```python
from build123d import *

# Parameters (mm, degrees)
BOSS_EXTRUDE1_DEPTH      = 30
SKETCH3_R                = 2.146244949
BOSS_EXTRUDE2_DEPTH      = 10
BOSS_EXTRUDE2_DEPTH_BACK = 104
SKETCH4_W                = 62.472603167
SKETCH4_H                = 24.76734243
CUT_EXTRUDE1_DEPTH       = 31
FILLET1_R                = 10
SKETCH5_R                = 0.76292284
BOSS_EXTRUDE3_DEPTH      = 30
SKETCH8_W                = 88.333137
SKETCH8_H                = 25.902143048
CUT_EXTRUDE2_DEPTH       = 5
SKETCH9_R                = 0.25
BOSS_EXTRUDE4_DEPTH      = 90


with BuildPart() as part:
    # Sketch1 → Boss-Extrude1 (new body)
    with BuildSketch(Plane(origin=(0, 0, 0), x_dir=(1, 0, 0), z_dir=(0, 1, 0))):
        Polygon((-80.330769327, 39.448145651), (-80.330769327, -54.366717098), (84.060412188, -54.366717098), (125.94717048, -7.459285723), (76.88802207, 39.448145651), align=None)
    extrude(amount=BOSS_EXTRUDE1_DEPTH)

    # Sketch2 → Cut-Revolve2 (revolve, cut)
    with BuildSketch(Plane(origin=(73.778167937, 0, 65.881422133), x_dir=(0.666061097, 0, -0.745897188), z_dir=(0.745897188, 0, 0.666061097))):
        with BuildLine():
            Line((32.647209403, 24.725169295), (66.605654017, 24.725169295))
            ThreePointArc((66.605654017, 24.725169295), (77.035151749, 14.295671563), (66.605654017, 3.866173832))
            Line((66.605654017, 3.866173832), (32.647209403, 3.866173832))
            ThreePointArc((32.647209403, 3.866173832), (22.217711672, 14.295671563), (32.647209403, 24.725169295))
        make_face()
    revolve(axis=Axis((125.94717048, 30, 7.459285723), (0, -1, 0)), mode=Mode.SUBTRACT)

    # Sketch3 → Boss-Extrude2 (add, two sides)
    with BuildSketch(Plane.XY.offset(54.366717098)) as boss_extrude2_sk:
        with Locations((-57.321321229, 15)):
            Circle(SKETCH3_R)
    extrude(amount=BOSS_EXTRUDE2_DEPTH)
    extrude(boss_extrude2_sk.sketch, amount=-BOSS_EXTRUDE2_DEPTH_BACK)

    # Sketch4 → Cut-Extrude1 (cut, through all)
    with BuildSketch(Plane(origin=(0, 30, 0), x_dir=(1, 0, 0), z_dir=(0, 1, 0))):
        with Locations((145.25317231, -8.435915945)):
            Rectangle(SKETCH4_W, SKETCH4_H)
    extrude(amount=-CUT_EXTRUDE1_DEPTH, mode=Mode.SUBTRACT)

    # Fillet1
    fillet1_edges = [part.edges().sort_by_distance(p)[0] for p in [
        (114.016870726, 1.933086916, 20.81958716),
        (114.016870726, 27.362584647, 20.81958716),
        (114.016870726, 1.933086916, -3.94775527),
        (114.016870726, 27.362584647, -3.94775527),
    ]]
    fillet(fillet1_edges, radius=FILLET1_R)

    # Sketch5 → Boss-Extrude3 (add)
    with BuildSketch(Plane(origin=(0, 30, 0), x_dir=(1, 0, 0), z_dir=(0, 1, 0))):
        with Locations((109.099187599, -8.665449149)):
            Circle(SKETCH5_R)
    extrude(amount=-BOSS_EXTRUDE3_DEPTH)

    # Sketch8 → Cut-Extrude2 (cut)
    with BuildSketch(Plane.ZY.offset(80.330769327)):
        with Locations((7.459285723, 15)):
            Rectangle(SKETCH8_W, SKETCH8_H)
    extrude(amount=-CUT_EXTRUDE2_DEPTH, mode=Mode.SUBTRACT)

    # Sketch9 → Boss-Extrude4 (add)
    with BuildSketch(Plane(origin=(0, 0, 51.625854223), x_dir=(-1, 0, 0), z_dir=(0, 0, -1))):
        with Locations((79.909462448, 27.17643451)):
            Circle(SKETCH9_R)
    extrude(amount=BOSS_EXTRUDE4_DEPTH)


solid = part.part
```
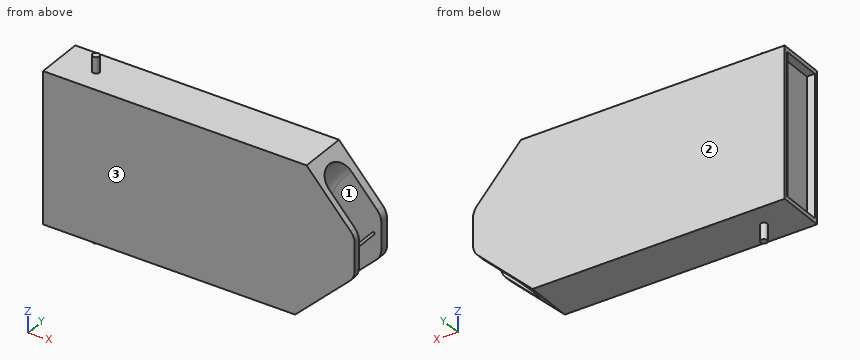
Geometry: final body of the model. Coordinates: model frame, mm. Face numbers are marked on the shaded views. Coordinates: 2 decimals unless noted, no trailing zeros. Order: outer loops, then holes, each group sorted by start corner. A loop starts at its lowest first (then second) coordinate and runs counter-clockwise, first axis right, second up.
Item 1: Draft query along Y for the marked faces 1, 2 and 3. Return one class per face: released by +Y, released by -Y, zero draft, split by the parting line, or undercut.
Answer:
face 1: undercut
face 2: released by +Y
face 3: released by -Y
Item 2: Section query B-B (x = 33). Output: boundary loops of the cut face in (y, z), then the cut area to 3 significant figures.
Answer:
outline: (0, -39.45) - (30, -39.45) - (30, 54.37) - (0, 54.37) - close
area: 2,810 mm2
Item 3: Section query A-A (y = 15). Output: boundary loops of the cut face in (x, z), then the cut area to 3 significant figures.
Answer:
outline: (-80.33, -39.45) - (-59.47, -39.45) - (-59.47, -49.63) - (-55.18, -49.63) - (-55.18, -39.45) - (76.89, -39.45) - (85.41, -31.3) arc R56.08 cw to (88.59, 49.29) - (84.06, 54.37) - (-55.18, 54.37) - (-55.18, 64.37) - (-59.47, 64.37) - (-59.47, 54.37) - (-80.33, 54.37) - (-80.33, 51.63) - (-75.33, 51.63) - (-75.33, -36.71) - (-80.33, -36.71) - close; circle Ø1.53 at (109.1, 8.67)
area: 14,300 mm2
Item 4: Contact query for flat-ended pins moving along their axis: P1, Ø8, axis at y = 7, z = -22.5, coming from the +X side; P2, Ø9, axis at x = -7.5, y = 17.5, coming from the +Z side; P3, Ø8, axis at y = 12.5, z = -13.5, coming from the +X side. Output: stop coordinate, or through.
Answer:
P1: stops at x = 97.21
P2: stops at z = 54.37
P3: stops at x = 76.34
Item 5: Material intervals for line 1 along Y through (x, z) = (99, 10); line 2 along Z through (x, y) = (-48, 22.5); line 3 along X through (y, z) = (27.25, 8.5), sorted ascending.
Answer:
line 1: y = 0 to 3.87, 24.73 to 30
line 2: z = -39.45 to 54.37
line 3: x = -80.15 to -79.67, -75.33 to 114.02
